from build123d import *

# Parameters (mm, degrees)
ESBO_O2_R                = 4.25
ESBO_O2_R_2              = 5.5
ESBO_O2_R_3              = 7
RESSALTO_EXTRUS_O2_DEPTH = 12
ESBO_O3_R                = 12
ESBO_O3_R_2              = 7
RESSALTO_EXTRUS_O3_DEPTH = 16
FILETE1_R                = 2


with BuildPart() as part:
    # Esboço2 → Ressalto-extrusão2 (new body)
    with BuildSketch(Plane(origin=(0, 0, 0), x_dir=(1, 0, 0), z_dir=(0, 1, 0))):
        with BuildLine():
            Line((-12.057610331, 26.374495883), (-43.708926586, 11.904485175))
            ThreePointArc((-43.708926586, 11.904485175), (-55.708926586, -0.095514825), (-43.708926586, -12.095514825))
            Line((-43.708926586, -12.095514825), (-11.925771547, -26.434371054))
            ThreePointArc((-11.925771547, -26.434371054), (0.12376622, -28.999735894), (12.150968312, -26.331615391))
            Line((12.150968312, -26.331615391), (43.35338336, -11.93297137))
            ThreePointArc((43.35338336, -11.93297137), (55.35338336, 0.06702863), (43.35338336, 12.06702863))
            Line((43.35338336, 12.06702863), (12.057610331, 26.374495883))
            ThreePointArc((12.057610331, 26.374495883), (0, 29), (-12.057610331, 26.374495883))
        make_face()
        with Locations(Location((-12.714926554, -12.082390656, 0), (0, 0, 90))):
            Circle(ESBO_O2_R, mode=Mode.SUBTRACT)
        with Locations(Location((12.285073446, -12.082390656, 0), (0, 0, 90))):
            Circle(ESBO_O2_R, mode=Mode.SUBTRACT)
        with Locations(Location((0, 0, 0), (0, 0, 90))):
            Circle(ESBO_O2_R_2, mode=Mode.SUBTRACT)
        with Locations(Location((-12.714788426, 12.000714001, 0), (0, 0, 90))):
            Circle(ESBO_O2_R, mode=Mode.SUBTRACT)
        with Locations(Location((12.285073446, 11.917609344, 0), (0, 0, 90))):
            Circle(ESBO_O2_R, mode=Mode.SUBTRACT)
        with Locations(Location((-43.708926586, -0.095514825, 0), (0, 0, 90))):
            Circle(ESBO_O2_R_3, mode=Mode.SUBTRACT)
        with Locations(Location((43.35338336, 0.06702863, 0), (0, 0, 90))):
            Circle(ESBO_O2_R_3, mode=Mode.SUBTRACT)
    extrude(amount=RESSALTO_EXTRUS_O2_DEPTH)

    # Esboço3 → Ressalto-extrusão3 (add)
    # profile 1 of 2: a face of its own
    with BuildSketch(Plane(origin=(0, 12, 0), x_dir=(1, 0, 0), z_dir=(0, 1, 0))):
        with Locations(Location((-43.708926586, -0.095514825, 0), (0, 0, 270))):
            Circle(ESBO_O3_R)
        with Locations(Location((-43.708926586, -0.095514825, 0), (0, 0, 90))):
            Circle(ESBO_O3_R_2, mode=Mode.SUBTRACT)
    # profile 2 of 2: a face of its own
    with BuildSketch(Plane(origin=(0, 12, 0), x_dir=(1, 0, 0), z_dir=(0, 1, 0))):
        with Locations(Location((43.35338336, 0.06702863, 0), (0, 0, 270))):
            Circle(ESBO_O3_R)
        with Locations(Location((43.35338336, 0.06702863, 0), (0, 0, 90))):
            Circle(ESBO_O3_R_2, mode=Mode.SUBTRACT)
    extrude(amount=RESSALTO_EXTRUS_O3_DEPTH)

    # Filete1
    filete1_edges = [part.edges().sort_by_distance(p)[0] for p in [
        (-43.708926586, 28, -11.904485175),
        (43.35338336, 28, -12.06702863),
    ]]
    fillet(filete1_edges, radius=FILETE1_R)


solid = part.part
Here's how the part is built. I have some questions about the finished solid (model axes, mm). A direction names the side the tool comes from. Coordinates: 2 decimals unless noted, no trailing zeros. Order: outer loops, then holes, each group sorted by start corner. A loop starts at its lowest first (then second) coordinate and runs counter-clockwise, first axis right, second up.
Item 1: If we section it at A-A on x = 0: List the corners of the cut face in (y, z) for me.
Result sheet:
outline: (0, -29) - (12, -29) - (12, -5.5) - (0, -5.5) - close; (0, 5.5) - (12, 5.5) - (12, 29) - (0, 29) - close
Item 2: If we section it at C-C on z = -15: List the corners of the cut face in (x, y) for me, plus the area to 3 significant figures.
Result sheet:
outline: (-36.94, 0) - (-15.73, 0) - (-15.73, 12) - (-36.94, 12) - close; (-9.7, 0) - (9.36, 0) - (9.36, 12) - (-9.7, 12) - close; (15.21, 0) - (36.94, 0) - (36.94, 12) - (15.21, 12) - close
area: 744 mm2
Item 3: If we section it at D-D on y = 6.75: List the corners of the cut face in (x, z) for me.
Result sheet:
outline: (-43.71, -11.9) - (-12.06, -26.37) arc R29 ccw to (12.06, -26.37) - (43.35, -12.07) arc R12 ccw to (43.35, 11.93) - (12.15, 26.33) arc R29 ccw to (-11.93, 26.43) - (-43.71, 12.1) arc R12 ccw to start; hole circle Ø14 at (-43.71, 0.1); hole circle Ø8.5 at (-12.71, -12); hole circle Ø8.5 at (-12.71, 12.08); hole circle Ø11 at (0, 0); hole circle Ø8.5 at (12.29, -11.92); hole circle Ø8.5 at (12.29, 12.08); hole circle Ø14 at (43.35, -0.07)
Item 4: For P1, Ø6, axis at x = 3, z = -6, coming from the +Y side; P2, Ø8, axis at y = 20, z = 18.5, coming from the -X side; P3, Ø5, axis at x = 16, y = 4.5, coming from the +Z side; P4, Ø3, axis at x = 32.5, y = 11.5, coming from the -Z side, each with a flat end and sliding along its axis, tell me the tip position at first contact or that it passes through.
Result sheet:
P1: stops at y = 12
P2: passes through
P3: stops at z = 25.71
P4: stops at z = -17.71
Item 5: I need wall thicknesses on line 1 (Z direction, x = -0.5, y = 11); line 2 (X direction, y = 7, z = 16); line 3 (Y direction, x = -3, z = 12.5). Which ranges of each line are inside material? Lowest first, please.
Result sheet:
line 1: z = -29 to -5.48, 5.48 to 29
line 2: x = -35.05 to -14.36, -11.07 to 10.64, 13.93 to 34.54
line 3: y = 0 to 12
Item 6: If we section it at B-B on y = 17.5: List the corners of the cut face in (x, z) for me, plus the area to 3 significant figures.
Result sheet:
outline: circle Ø24 at (-43.71, 0.1); circle Ø24 at (43.35, -0.07); hole circle Ø14 at (-43.71, 0.1); hole circle Ø14 at (43.35, -0.07)
area: 597 mm2
Item 7: If we mould it in two halves opening along Z, with no side actions, what happens to faces 3 (the face through (8.7, 5.9, 9.8)), 4 (the face through (0, 6, 29)), 5 (the face through (0, 6, -29))? For each: +Z half, -Z half, draft (parallel to the pull), parting line (faces both ways), or undercut.
Result sheet:
face 3: undercut
face 4: +Z half
face 5: -Z half
Item 8: For faces 1 (the face through (5.37, 5.92, 1.19)), 2 (the face through (-55.683, 9.929, -0.696)), which set-ups out of +Z, -Z, +X, -X, +Y, -Y let a thin tool reach every point of the face, with its end or its side?
Result sheet:
face 1: +Y, -Y
face 2: +Y
